The listing builds one solid part. Answer for the finished solid, in the listing's coordinates (mm). Face numbers are marked on the shaded views. A direction names the side the tool comes from. Coordinates: 2 decimals unless noted, no trailing zeros. Order: outer loops, then holes, each group sorted by start corner. A loop starts at its lowest first (then second) coordinate and runs counter-clockwise, first axis right, second up. Notation, with made-up numbers: (50, 1) -> (103, 1) arc R6 ccw to (103, 6) -> close; hole circle Ø2 at (83, 1.5). An arc over 180 degrees is marked (long way). Return JSON: item names as keys, results as strings.
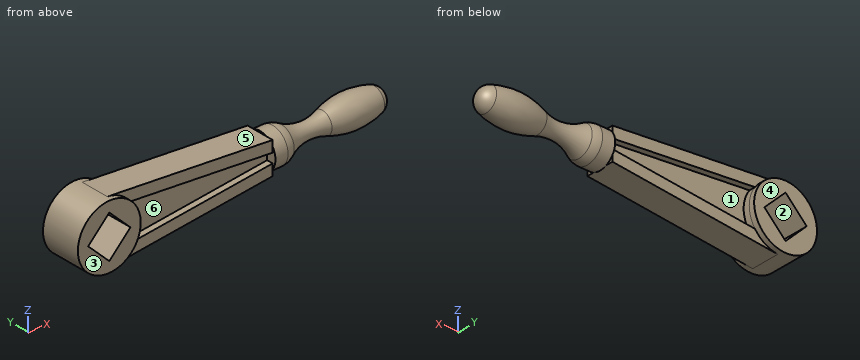
from build123d import *
from build123d.topology import SkipClean

# Parameters (mm, degrees)
SKETCH_1_R          = 20
EXTRUDE_1_DEPTH     = 12.5
EXTRUDE_2_DEPTH     = 9
CUT_EXTRUDE_START   = 5
CUT_EXTRUDE_1_DEPTH = 4
CUT_EXTRUDE_START_2 = -9
CUT_EXTRUDE_2_DEPTH = 4


with BuildPart() as part:
    # 草图1 → 凸台-拉伸1 (new, symmetric)
    with BuildSketch(Plane(origin=(0, 0, 0), x_dir=(1, 0, 0), z_dir=(0, 1, 0))):
        with Locations(Location((0, 0, 0), (0, 0, 270))):
            Circle(SKETCH_1_R)
        Polygon((0, 13.435028843), (13.435028843, 0), (0, -13.435028843), (-13.435028843, 0), align=None, mode=Mode.SUBTRACT)
    extrude(amount=EXTRUDE_1_DEPTH, both=True)

    # 草图2 → 凸台-拉伸2 (add, symmetric)
    with BuildSketch(Plane(origin=(0, 0, 0), x_dir=(1, 0, 0), z_dir=(0, 1, 0))):
        with BuildLine():
            ThreePointArc((1.877412327, 19.911688099), (14.791014951, 13.462016072), (20, 0))
            Line((20, 0), (107, 0))
            Line((107, 0), (107, 10))
            Line((107, 10), (1.877412327, 19.911688099))
        make_face()
        with BuildLine():
            Line((107, 0), (20, 0))
            ThreePointArc((20, 0), (14.791014951, -13.462016072), (1.877412327, -19.911688099))
            Line((1.877412327, -19.911688099), (107, -10))
            Line((107, -10), (107, 0))
        make_face()
    extrude(amount=EXTRUDE_2_DEPTH, both=True)

    # 草图3 → 切除-拉伸1 (cut)
    with SkipClean():  # the faces are left unmerged after this step: merging them gives an invalid solid
        with BuildSketch(Plane(origin=(0, 0, 0), x_dir=(1, 0, 0), z_dir=(0, 1, 0)).offset(CUT_EXTRUDE_START)):
            with BuildLine():
                Line((107, 2.968953747), (16.351890932, 11.515887415))
                ThreePointArc((16.351890932, 11.515887415), (20, 0), (16.351890932, -11.515887415))
                Line((16.351890932, -11.515887415), (107, -2.968953747))
                Line((107, -2.968953747), (107, 2.968953747))
            make_face()
        extrude(amount=CUT_EXTRUDE_1_DEPTH, mode=Mode.SUBTRACT)

    # 草图3<2> → 切除-拉伸2 (cut)
    with SkipClean():  # the faces are left unmerged after this step: merging them gives an invalid solid
        with BuildSketch(Plane(origin=(0, 0, 0), x_dir=(1, 0, 0), z_dir=(0, 1, 0)).offset(CUT_EXTRUDE_START_2)):
            with BuildLine():
                Line((107, 2.968953747), (16.351890932, 11.515887415))
                ThreePointArc((16.351890932, 11.515887415), (20, 0), (16.351890932, -11.515887415))
                Line((16.351890932, -11.515887415), (107, -2.968953747))
                Line((107, -2.968953747), (107, 2.968953747))
            make_face()
        extrude(amount=CUT_EXTRUDE_2_DEPTH, mode=Mode.SUBTRACT)

    # 草图4 → 旋转1 (revolve)
    with SkipClean():  # the faces are left unmerged after this step: merging them gives an invalid solid
        with BuildSketch(Plane(origin=(0, 0, 0), x_dir=(1, 0, 0), z_dir=(0, 1, 0)), mode=Mode.PRIVATE) as revolve_1_sk:
            with BuildLine():
                Line((107, 0), (107, 11))
                Line((107, 11), (115, 11))
                ThreePointArc((115, 11), (117.753651476, 10.613397087), (120.294389016, 9.483480709))
                ThreePointArc((120.294389016, 9.483480709), (133.180287907, 5.08402529), (146.683629362, 6.833701774))
                ThreePointArc((146.683629362, 6.833701774), (162.995301682, 9.985635116), (179.439285424, 7.619047619))
                ThreePointArc((179.439285424, 7.619047619), (183.461976609, 4.716233487), (185, 0))
                Line((185, 0), (107, 0))
            make_face()
        revolve(revolve_1_sk.sketch.rotate(Axis((0, 0, 0), (1, 0, 0)), 180), axis=Axis((0, 0, 0), (1, 0, 0)))


solid = part.part
1. The part is cut by section C-C on x = 81. Give the vertices of the cut face in (y, z), and give its area (3 significant figures).
Answer block:
{"outline": "(-9, -12.45) -> (9, -12.45) -> (9, -5.42) -> (5, -5.42) -> (5, 5.42) -> (9, 5.42) -> (9, 12.45) -> (-9, 12.45) -> (-9, 5.42) -> (-5, 5.42) -> (-5, -5.42) -> (-9, -5.42) -> close", "area": "362 mm2"}
2. Each of these flat-tipped pins is pushed along its axis until it touches: pin 1 Ø1.5 at (x, y) = (101.5, -5) entering from -Z; pin 2 Ø3 at (y, z) = (-6.5, 1) entering from +X; pin 3 Ø5 at (x, y) = (4, -8.5) entering from -Z. Where does it stop, or does it pass through?
Answer block:
{"pin 1": "stops at z = -10.59", "pin 2": "stops at x = 183.18", "pin 3": "stops at z = -19.94"}
3. Consider line 1 (Z direction, x = 71, y = 6); line 2 (Y direction, x = 59, z = -13.5); line 3 (Y direction, x = 48, z = 0). Determine where each line is inside the solid, lowest interval first. Write a range as from..to.
Answer block:
{"line 1": "z = -13.39..-6.36, 6.36..13.39", "line 2": "y = -9..9", "line 3": "y = -5..5"}
4. Determine the mould class of the marked faces 4, 5 and 6 for opening direction Z: pulls with the +Z half, pulls with the -Z half, needs draft (parallel to the pull), parting line crosses it, or undercut.
Answer block:
{"face 4": "needs draft", "face 5": "pulls with the +Z half", "face 6": "undercut"}
5. For the marked faces 1, 2 and 3, determine the directions among +Z, -Z, +X, -X, +Y, -Y from which every point of the face is accessible in a straight line to the end or side of a thin tool.
Answer block:
{"face 1": "+Y", "face 2": "+Y, -Y", "face 3": "+Z, -Z, +X, -X, -Y"}
6. The part is cut by section A-A on x = -4.5. Give the vertices of the cut face in (y, z), and give its area (3 significant figures).
Answer block:
{"outline": "(-12.5, -19.49) -> (12.5, -19.49) -> (12.5, -8.94) -> (-12.5, -8.94) -> close; (-12.5, 8.94) -> (12.5, 8.94) -> (12.5, 19.49) -> (-12.5, 19.49) -> close", "area": "528 mm2"}
7. The part is cut by section B-B on x = 56. Give the vertices of the cut face in (y, z).
Answer block:
{"outline": "(-9, -14.81) -> (9, -14.81) -> (9, -7.78) -> (5, -7.78) -> (5, 7.78) -> (9, 7.78) -> (9, 14.81) -> (-9, 14.81) -> (-9, 7.78) -> (-5, 7.78) -> (-5, -7.78) -> (-9, -7.78) -> close"}
